Part model, mm, in its own coordinate system. Face numbers are marked on the shaded views. A direction names the side the tool comes from. Round coordinates to 2 decimals unless told otherwise and drop trailing zeros. Write each loop counter-clockwise with the first axis right and the second up, starting at its lowest first coordinate (ties: lowest second). Pieces come first, ordered by that corner, then holes. Notation, with made-up numbers: M 86.5,-11.5 L 112.5,-11.5 A29 ccw 112.5,9.5 Z; hole C -39,15.5 d3. An arc over 180 degrees is marked long. Use a Markdown table: item, result. Add a question column.
1) Slice it at B-B on x = 5. Write the cut outline in (y, z) (3 decimals), plus the area to 3 significant figures.
2) Drop flat-ended pins along their axis: P1, Ø8, axis at x = -41, y = -7.5, coming from the -Z side; P2, Ø5, axis at x = -44, z = 56, coming from the -Y side. Give the stop position or say it passes through.
3) Slice it at C-C on y = -5.5. Write the cut outline in (x, z), plus the area to 3 significant figures.
4) Which spindle directions (+Z, -Z, +X, -X, +Y, -Y) get a long thin tool onto all of the face, cutting with end or side? Do the marked faces 1 and 2. Say none if no direction does.
5) Wall check: probe 1 along Z at (x, y) = (94, -7); probe 2 along Y at (x, z) = (78, 58); probe 3 along Z at (x, y) = (-59.5, -1). Give the ranges that are in metal, low to high.
6) Slice it at A-A on z = 42.5. Write the cut outline in (x, y), plus the area to 3 significant figures.
7) Slice it at D-D on z = -2.5. Write the cut outline in (x, y), plus the area to 3 significant figures.
```python
from build123d import *

# Parameters (mm, degrees)
SKETCH1_W                    = 189.8572
SKETCH1_H                    = 175.514
BASE_FLANGE1_DEPTH           = 2.3622
EDGE_FLANGE4_STRIP_W         = 11.0744
EDGE_FLANGE4_STRIP_H         = 2.3622
EDGE_FLANGE4_STRIP_CUT_DEPTH = 189.8572
EDGE_FLANGE4_DEPTH           = 189.8572
CUT_EXTRUDE1_DEPTH           = 145.352665205
CUT_EXTRUDE5_REACH           = 151.669
SKETCH41_R                   = 2.4765
CUT_EXTRUDE6_REACH           = 138.891
SKETCH42_R                   = 2.413
SKETCH42_R_2                 = 2.4765
CUT_EXTRUDE7_REACH           = 138.891
SKETCH43_R                   = 4.7625


# Sheet-metal steps are written as plain solids
with BuildPart() as part:
    # Sketch1 → Base-Flange1 (new body)
    with BuildSketch(Plane(origin=(0, 0, 0), x_dir=(1, 0, 0), z_dir=(0, 1, 0))):
        with Locations((12.6128, 7.08)):
            Rectangle(SKETCH1_W, SKETCH1_H)
    extrude(amount=-BASE_FLANGE1_DEPTH)

    # Edge-Flange4 strip (across the edge) → Edge-Flange4 strip cut (cut)
    with BuildSketch(Plane(origin=(107.5414, -2.3622, 80.677), x_dir=(0, 0, -1), z_dir=(-1, 0, 0))):
        with Locations((-4.7244, -1.1811)):
            Rectangle(EDGE_FLANGE4_STRIP_W, EDGE_FLANGE4_STRIP_H)
    extrude(amount=EDGE_FLANGE4_STRIP_CUT_DEPTH, mode=Mode.SUBTRACT)

    # Edge-Flange4 section (across the edge) → Edge-Flange4 (add)
    with BuildSketch(Plane(origin=(107.5414, -2.3622, 80.677), x_dir=(0, 0, -1), z_dir=(-1, 0, 0))):
        with BuildLine():
            Line((-2.3622, 0.8128), (-2.3622, 16.6878))
            Line((-2.3622, 16.6878), (0, 16.6878))
            Line((0, 16.6878), (0, 0.8128))
            ThreePointArc((0, 0.8128), (0.238063608, 0.238063608), (0.8128, 0))
            Line((0.8128, 0), (0.8128, -2.3622))
            ThreePointArc((0.8128, -2.3622), (-1.43226403, -1.43226403), (-2.3622, 0.8128))
        make_face()
    extrude(amount=EDGE_FLANGE4_DEPTH)

    # Sketch36 → Cut-Extrude1 (cut, through all)
    with BuildSketch(Plane.XZ.offset(2.3622)):
        Polygon((20.98856689, -21.6596), (-82.3158, -21.6596), (-82.3158, -94.837), (107.5414, -94.837), (107.5414, 50.96685034), align=None)
    extrude(amount=-CUT_EXTRUDE1_DEPTH, mode=Mode.SUBTRACT)

    # Sketch41 → Cut-Extrude5 (cut, up to next)
    with BuildSketch(Plane(origin=(0, 0, 80.677), x_dir=(-1, 0, 0), z_dir=(0, 0, -1)), mode=Mode.PRIVATE) as cut_extrude5_sk1:
        with Locations(Location((-88.8128, -11.1125, 0), (0, 0, 90))):
            Circle(SKETCH41_R)
    cut_extrude5_tool1 = extrude(cut_extrude5_sk1.sketch, amount=-CUT_EXTRUDE5_REACH, mode=Mode.PRIVATE) & part.part
    # Sketch41 → Cut-Extrude5 (cut, up to next)
    with BuildSketch(Plane(origin=(0, 0, 80.677), x_dir=(-1, 0, 0), z_dir=(0, 0, -1)), mode=Mode.PRIVATE) as cut_extrude5_sk2:
        with Locations(Location((-63.4128, -11.1125, 0), (0, 0, 90))):
            Circle(SKETCH41_R)
    cut_extrude5_tool2 = extrude(cut_extrude5_sk2.sketch, amount=-CUT_EXTRUDE5_REACH, mode=Mode.PRIVATE) & part.part
    # Sketch41 → Cut-Extrude5 (cut, up to next)
    with BuildSketch(Plane(origin=(0, 0, 80.677), x_dir=(-1, 0, 0), z_dir=(0, 0, -1)), mode=Mode.PRIVATE) as cut_extrude5_sk3:
        with Locations(Location((-38.0128, -11.1125, 0), (0, 0, 90))):
            Circle(SKETCH41_R)
    cut_extrude5_tool3 = extrude(cut_extrude5_sk3.sketch, amount=-CUT_EXTRUDE5_REACH, mode=Mode.PRIVATE) & part.part
    # Sketch41 → Cut-Extrude5 (cut, up to next)
    with BuildSketch(Plane(origin=(0, 0, 80.677), x_dir=(-1, 0, 0), z_dir=(0, 0, -1)), mode=Mode.PRIVATE) as cut_extrude5_sk4:
        with Locations(Location((-12.6128, -11.1125, 0), (0, 0, 90))):
            Circle(SKETCH41_R)
    cut_extrude5_tool4 = extrude(cut_extrude5_sk4.sketch, amount=-CUT_EXTRUDE5_REACH, mode=Mode.PRIVATE) & part.part
    # Sketch41 → Cut-Extrude5 (cut, up to next)
    with BuildSketch(Plane(origin=(0, 0, 80.677), x_dir=(-1, 0, 0), z_dir=(0, 0, -1)), mode=Mode.PRIVATE) as cut_extrude5_sk5:
        with Locations(Location((12.7872, -11.1125, 0), (0, 0, 90))):
            Circle(SKETCH41_R)
    cut_extrude5_tool5 = extrude(cut_extrude5_sk5.sketch, amount=-CUT_EXTRUDE5_REACH, mode=Mode.PRIVATE) & part.part
    # Sketch41 → Cut-Extrude5 (cut, up to next)
    with BuildSketch(Plane(origin=(0, 0, 80.677), x_dir=(-1, 0, 0), z_dir=(0, 0, -1)), mode=Mode.PRIVATE) as cut_extrude5_sk6:
        with Locations(Location((38.1872, -11.1125, 0), (0, 0, 90))):
            Circle(SKETCH41_R)
    cut_extrude5_tool6 = extrude(cut_extrude5_sk6.sketch, amount=-CUT_EXTRUDE5_REACH, mode=Mode.PRIVATE) & part.part
    # Sketch41 → Cut-Extrude5 (cut, up to next)
    with BuildSketch(Plane(origin=(0, 0, 80.677), x_dir=(-1, 0, 0), z_dir=(0, 0, -1)), mode=Mode.PRIVATE) as cut_extrude5_sk7:
        with Locations(Location((63.5872, -11.1125, 0), (0, 0, 90))):
            Circle(SKETCH41_R)
    cut_extrude5_tool7 = extrude(cut_extrude5_sk7.sketch, amount=-CUT_EXTRUDE5_REACH, mode=Mode.PRIVATE) & part.part
    add(cut_extrude5_tool1.solids().sort_by_distance((88.8128, -11.1125, 80.677))[0], mode=Mode.SUBTRACT)
    add(cut_extrude5_tool2.solids().sort_by_distance((63.4128, -11.1125, 80.677))[0], mode=Mode.SUBTRACT)
    add(cut_extrude5_tool3.solids().sort_by_distance((38.0128, -11.1125, 80.677))[0], mode=Mode.SUBTRACT)
    add(cut_extrude5_tool4.solids().sort_by_distance((12.6128, -11.1125, 80.677))[0], mode=Mode.SUBTRACT)
    add(cut_extrude5_tool5.solids().sort_by_distance((-12.7872, -11.1125, 80.677))[0], mode=Mode.SUBTRACT)
    add(cut_extrude5_tool6.solids().sort_by_distance((-38.1872, -11.1125, 80.677))[0], mode=Mode.SUBTRACT)
    add(cut_extrude5_tool7.solids().sort_by_distance((-63.5872, -11.1125, 80.677))[0], mode=Mode.SUBTRACT)

    # Sketch42 → Cut-Extrude6 (cut, up to next)
    with BuildSketch(Plane.XZ.offset(2.3622), mode=Mode.PRIVATE) as cut_extrude6_sk1:
        with Locations(Location((-74.3402, -8.2596, 0), (0, 0, 270))):
            Circle(SKETCH42_R)
    cut_extrude6_tool1 = extrude(cut_extrude6_sk1.sketch, amount=-CUT_EXTRUDE6_REACH, mode=Mode.PRIVATE) & part.part
    # Sketch42 → Cut-Extrude6 (cut, up to next)
    with BuildSketch(Plane.XZ.offset(2.3622), mode=Mode.PRIVATE) as cut_extrude6_sk2:
        with Locations(Location((-74.3402, 17.1404, 0), (0, 0, 270))):
            Circle(SKETCH42_R)
    cut_extrude6_tool2 = extrude(cut_extrude6_sk2.sketch, amount=-CUT_EXTRUDE6_REACH, mode=Mode.PRIVATE) & part.part
    # Sketch42 → Cut-Extrude6 (cut, up to next)
    with BuildSketch(Plane.XZ.offset(2.3622), mode=Mode.PRIVATE) as cut_extrude6_sk3:
        with Locations(Location((-74.3402, 42.5404, 0), (0, 0, 270))):
            Circle(SKETCH42_R)
    cut_extrude6_tool3 = extrude(cut_extrude6_sk3.sketch, amount=-CUT_EXTRUDE6_REACH, mode=Mode.PRIVATE) & part.part
    # Sketch42 → Cut-Extrude6 (cut, up to next)
    with BuildSketch(Plane.XZ.offset(2.3622), mode=Mode.PRIVATE) as cut_extrude6_sk4:
        with Locations(Location((-74.3402, 67.9404, 0), (0, 0, 270))):
            Circle(SKETCH42_R)
    cut_extrude6_tool4 = extrude(cut_extrude6_sk4.sketch, amount=-CUT_EXTRUDE6_REACH, mode=Mode.PRIVATE) & part.part
    # Sketch42 → Cut-Extrude6 (cut, up to next)
    with BuildSketch(Plane.XZ.offset(2.3622), mode=Mode.PRIVATE) as cut_extrude6_sk5:
        with Locations(Location((99.5658, 59.3664, 0), (0, 0, 270))):
            Circle(SKETCH42_R_2)
    cut_extrude6_tool5 = extrude(cut_extrude6_sk5.sketch, amount=-CUT_EXTRUDE6_REACH, mode=Mode.PRIVATE) & part.part
    # Sketch42 → Cut-Extrude6 (cut, up to next)
    with BuildSketch(Plane.XZ.offset(2.3622), mode=Mode.PRIVATE) as cut_extrude6_sk6:
        with Locations(Location((99.5658, 72.0664, 0), (0, 0, 270))):
            Circle(SKETCH42_R_2)
    cut_extrude6_tool6 = extrude(cut_extrude6_sk6.sketch, amount=-CUT_EXTRUDE6_REACH, mode=Mode.PRIVATE) & part.part
    add(cut_extrude6_tool1.solids().sort_by_distance((-74.3402, -2.3622, -8.2596))[0], mode=Mode.SUBTRACT)
    add(cut_extrude6_tool2.solids().sort_by_distance((-74.3402, -2.3622, 17.1404))[0], mode=Mode.SUBTRACT)
    add(cut_extrude6_tool3.solids().sort_by_distance((-74.3402, -2.3622, 42.5404))[0], mode=Mode.SUBTRACT)
    add(cut_extrude6_tool4.solids().sort_by_distance((-74.3402, -2.3622, 67.9404))[0], mode=Mode.SUBTRACT)
    add(cut_extrude6_tool5.solids().sort_by_distance((99.5658, -2.3622, 59.3664))[0], mode=Mode.SUBTRACT)
    add(cut_extrude6_tool6.solids().sort_by_distance((99.5658, -2.3622, 72.0664))[0], mode=Mode.SUBTRACT)

    # Sketch43 → Cut-Extrude7 (cut, up to next)
    with BuildSketch(Plane.XZ.offset(2.3622), mode=Mode.PRIVATE) as cut_extrude7_sk1:
        with Locations(Location((-2.9408, 16.4404, 0), (0, 0, 270))):
            Circle(SKETCH43_R)
    cut_extrude7_tool1 = extrude(cut_extrude7_sk1.sketch, amount=-CUT_EXTRUDE7_REACH, mode=Mode.PRIVATE) & part.part
    add(cut_extrude7_tool1.solids().sort_by_distance((-2.9408, -2.3622, 16.4404))[0], mode=Mode.SUBTRACT)


solid = part.part
```
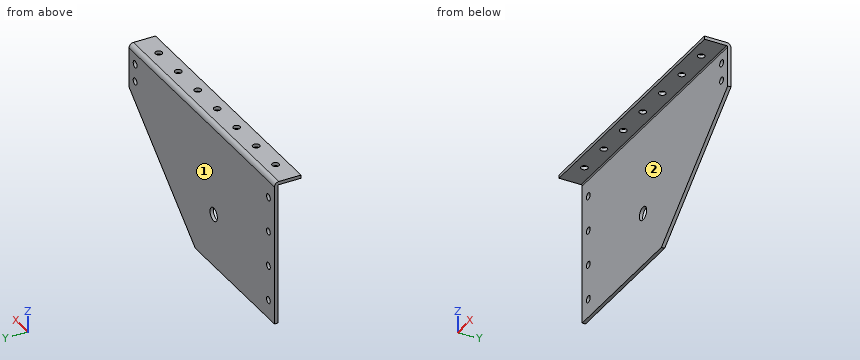
Entries:
| question | item | result |
|---|---|---|
| 1 | outline | M -19.05,80.677 L -3.175,80.677 A0.813 cw -2.362,79.864 L -2.362,-21.66 L 0,-21.66 L 0,79.864 A3.175 ccw -3.175,83.039 L -19.05,83.039 Z |
| 1 | area | 285 mm^2 |
| 2 | P1 | stops at z = 80.68 |
| 2 | P2 | stops at y = -2.36 |
| 3 | outline | M -82.32,80.68 L 107.54,80.68 L 107.54,83.04 L -82.32,83.04 Z |
| 3 | area | 448 mm^2 |
| 4 | face 1 | +Z, -Z, +X, -X, +Y |
| 4 | face 2 | -Z, +X, -X, -Y |
| 5 | probe 1 | z = 80.68 to 83.04 |
| 5 | probe 2 | y = -2.36 to 0 |
| 5 | probe 3 | z = -21.66 to 82.18 |
| 6 | outline | M -82.32,-2.36 L -76.75,-2.36 L -76.75,0 L -82.32,0 Z; M -71.93,-2.36 L 97.45,-2.36 L 97.45,0 L -71.93,0 Z |
| 6 | area | 413 mm^2 |
| 7 | outline | M -82.32,-2.36 L 43.82,-2.36 L 43.82,0 L -82.32,0 Z |
| 7 | area | 298 mm^2 |
